from build123d import *

# Parameters (mm, degrees)
SKETCH_W     = 2
SKETCH_H     = 46.5
SKETCH_W_2   = 38.408486
SKETCH_H_2   = 2
PAD_DEPTH    = 63.57
POCKET_DEPTH = 48.305243


with BuildPart() as part:
    # Sketch → Pad (new body)
    with BuildSketch(Plane.XZ):
        Polygon((-21.204243, 0), (-21.204243, 1.93), (-23.704243, 1.93), (-23.704243, 0), (-25.134243, 0), (-27.1, 1.965757), (-27.1, 7.655757), (-25.134243, 9.621514), (-23.704243, 9.621514), (-23.704243, 7.691514), (-21.204243, 7.691514), (-21.204243, 9.62), (-19.204243, 9.62), (-19.204243, 0), align=None)
        Polygon((19.204243, 9.62), (19.204243, 0), (21.204243, 0), (21.204243, 1.93), (23.704243, 1.93), (23.704243, 0), (25.134243, 0), (27.1, 1.965757), (27.1, 7.655757), (25.134243, 9.621514), (23.704243, 9.621514), (23.704243, 7.691514), (21.204243, 7.691514), (21.204243, 9.62), align=None)
        with Locations((20.204243, 32.87)):
            Rectangle(SKETCH_W, SKETCH_H)
        with Locations((-20.204243, 32.87)):
            Rectangle(SKETCH_W, SKETCH_H)
        with Locations((0, 55.12)):
            Rectangle(SKETCH_W_2, SKETCH_H_2)
    extrude(amount=PAD_DEPTH)

    # Sketch001 (on Face26 of Pad) → Pocket (cut, through all)
    with BuildSketch(Plane(origin=(-21.204243, 0, 0), x_dir=(0, 0, -1), z_dir=(-1, 0, 0))):
        Polygon((-19.62, 0), (-56.62, 64.08588), (-56.62, 0), align=None)
    extrude(amount=-POCKET_DEPTH, mode=Mode.SUBTRACT)


solid = part.part
Could you check a few things on this model? Use its own coordinates, in mm. A direction names the side the tool comes from. Give positions to 0.01 mm unless a question says otherwise; leave off trailing zeros. Order: outer loops, then holes, each group sorted by start corner. A loop starts at its lowest first (then second) coordinate and runs counter-clockwise, first axis right, second up. Notation, with made-up numbers: (49, 18.5) - (74, 18.5) arc R12 ccw to (74, 36.5) - close; hole circle Ø10 at (25.25, -40). An arc over 180 degrees is marked (long way). Return JSON: item names as keys, results as strings. Group by question number.
Q1. Suppose I cut it at B-B, the plane y = -16. Please give me the cut outline in (x, z).
Q2. Suppose I cut it at A-A, the plane z = 15. Please give me the cut outline in (x, y).
Q3. Suppose I cut it at D-D, the plane x = -0.5. Please give me the cut outline in (y, z), and give its area (3 significant figures).
Q4. Thinking about a two-plate mould opening in X: for faces 1 (the face through (-27.1, -31, 5)), 2 (the face through (19.204, -38, 21)), 3 (the face through (27.1, -31, 5)), which applies, pulls with the +X half, pulls with the -X half, needs draft (parallel to the pull), parting line crosses it, or undercut?
Q5. Which directions (+Z, -Z, +X, -X, +Y, -Y) give clear straight access to the entire face, cutting with the end or side of a thin tool? Please do faces 4 (the face through (22, -31, 1.93)), 5 (the face through (-26.103, -31.34, 0.969)), 6 (the face through (-22, -31, 7.692)).
Q6. Please list where these lines run through material, in increasing order: line 1 along X through (y, z) = (-12, 15); line 2 along X through (y, z) = (-12, 5); line 3 along Z through (x, y) = (-22, -9). Write a range as [from, to].
Q7. Suppose I cut it at C-C, the plane z = 5.5. Please give me the cut outline in (x, y), and give its area (3 significant figures).
Q8. Will these pins go through, and if not, where does the flat tip stop? pin 1 Ø1.2 at (x, y) = (22.5, -46) entering from +Z; pin 2 Ø14.5 at (y, z) = (-32.5, 42.5) entering from +X; pin 3 Ø1.2 at (x, y) = (-22.5, -42) entering from -Z.
Resolved:
{
 "1": {"outline": "(-27.1, 1.97) - (-25.13, 0) - (-23.7, 0) - (-23.7, 1.93) - (-21.2, 1.93) - (-21.2, 0) - (-19.2, 0) - (-19.2, 28.86) - (-21.2, 28.86) - (-21.2, 7.69) - (-23.7, 7.69) - (-23.7, 9.62) - (-25.13, 9.62) - (-27.1, 7.66) - close; (19.2, 0) - (21.2, 0) - (21.2, 1.93) - (23.7, 1.93) - (23.7, 0) - (25.13, 0) - (27.1, 1.97) - (27.1, 7.66) - (25.13, 9.62) - (23.7, 9.62) - (23.7, 7.69) - (21.2, 7.69) - (21.2, 28.86) - (19.2, 28.86) - close"},
 "2": {"outline": "(-21.2, -63.57) - (-19.2, -63.57) - (-19.2, 0) - (-21.2, 0) - close; (19.2, -63.57) - (21.2, -63.57) - (21.2, 0) - (19.2, 0) - close"},
 "3": {"outline": "(-63.57, 54.12) - (-59.76, 54.12) - (-63.22, 56.12) - (-63.57, 56.12) - close", "area": "4.16 mm2"},
 "4": {"face 1": "pulls with the -X half", "face 2": "undercut", "face 3": "pulls with the +X half"},
 "5": {"face 4": "-Z, +Y, -Y", "face 5": "-Z, -X, +Y, -Y", "face 6": "+Z, +Y, -Y"},
 "6": {"line 1": "x = [-21.2, -19.2], [19.2, 21.2]", "line 2": "x = [-27.1, -19.2], [19.2, 27.1]", "line 3": "z = [1.93, 7.69]"},
 "7": {"outline": "(-27.1, -63.57) - (-19.2, -63.57) - (-19.2, 0) - (-27.1, 0) - close; (19.2, -63.57) - (27.1, -63.57) - (27.1, 0) - (19.2, 0) - close", "area": "1,000 mm2"},
 "8": {"pin 1": "stops at z = 7.69", "pin 2": "stops at x = 21.2", "pin 3": "stops at z = 1.93"}
}
